```python
from build123d import *

# Parameters (mm, degrees)
EXTRUDE_1_DEPTH = 4


with BuildPart() as part:
    # 草图1 → 凸台-拉伸1 (new, symmetric)
    with BuildSketch(Plane.XY):
        with BuildLine():
            Line((5.85, -6), (-5.85, -6))
            ThreePointArc((-5.85, -6), (-6.557106781, -5.707106781), (-6.85, -5))
            Line((-6.85, -5), (-6.85, 0))
            Line((-6.85, 0), (6.85, 0))
            Line((6.85, 0), (6.85, -5))
            ThreePointArc((6.85, -5), (6.557106781, -5.707106781), (5.85, -6))
        make_face()
    extrude(amount=EXTRUDE_1_DEPTH, both=True)

    # 草图3 → 旋转1 (revolve)
    with BuildSketch(Plane.XY, mode=Mode.PRIVATE) as revolve_1_sk:
        Polygon((0, 25), (0, 0), (4, 0), (4, 2), (3.475115443, 2), (4, 2.320860647), (3.3, 2.748768937), (4, 3.176677227), (3.3, 3.604585516), (4, 4.032493806), (3.3, 4.460402096), (4, 4.888310385), (3.3, 5.316218675), (4, 5.744126965), (3.3, 6.172035254), (4, 6.599943544), (3.3, 7.027851834), (4, 7.455760123), (3.3, 7.883668413), (4, 8.311576703), (3.3, 8.739484992), (4, 9.167393282), (3.3, 9.595301572), (4, 10.023209861), (3.3, 10.451118151), (4, 10.879026441), (3.3, 11.30693473), (4, 11.73484302), (3.3, 12.16275131), (4, 12.590659599), (3.3, 13.018567889), (4, 13.446476179), (3.3, 13.874384469), (4, 14.302292758), (3.3, 14.730201048), (4, 15.158109338), (3.3, 15.586017627), (4, 16.013925917), (3.3, 16.441834207), (4, 16.869742496), (3.3, 17.297650786), (4, 17.725559076), (3.3, 18.153467365), (4, 18.581375655), (3.3, 19.009283945), (4, 19.437192234), (3.3, 19.865100524), (4, 20.293008814), (3.3, 20.720917103), (4, 21.148825393), (3.3, 21.576733683), (4, 22.004641972), (3.3, 22.432550262), (4, 22.860458552), (3.3, 23.288366841), (4, 23.716275131), (3.3, 24.144183421), (4, 24.57209171), (3.3, 25), align=None)
    revolve(revolve_1_sk.sketch.rotate(Axis((0, 25, 0), (0, 1, 0)), 270), axis=Axis((0, 25, 0), (0, 1, 0)))


solid = part.part
```
For this review, take the finished solid that the model builds, in its own axes (mm). Give positions to 0.01 mm unless a question says otherwise; leave off trailing zeros. Write each loop counter-clockwise with the first axis right and the second up, starting at its lowest first coordinate (ties: lowest second). Pieces come first, ordered by that corner, then holes.
Item 1: Take a section at A-A (x = 5). Give the boundary of the cut face in (y, z), and give its area (3 significant figures).
Item 2: Wall thickness on probe 1 along Y at (x, z) = (5.5, -3); probe 2 along Z at (x, y) = (-0.75, 9); probe 3 along Z at (x, y) = (2.5, 11): over which ranges is each line inside the solid? List them lowest first.
Item 3: Insertion check: P1, Ø6, axis at x = -3, y = 14, coming from the -Z side; P2, Ø1, axis at y = 6, z = 3, coming from the +X side; P3, Ø4, axis at y = 14, z = 2, coming from the -X side; P4, Ø1, axis at x = -3, y = 2, coming from the +Z side. Each pin has a flat end and moves straight along its axis. Give the tip position at first contact, or say it passes through.
Established:
1. outline: (-6, -4) - (0, -4) - (0, 4) - (-6, 4) - close
1. area: 48.0 mm2
2. probe 1: y = -6 to 0
2. probe 2: z = -3.65 to 3.65
2. probe 3: z = -2.86 to 2.86
3. P1: stops at z = -4
3. P2: stops at x = 3.06
3. P3: stops at x = -4
3. P4: stops at z = 3.12
